Input: part model. Units: mm. Frame: model coordinates. Face numbers are marked on the shaded views. A direction names the side the tool comes from. Give positions to 0.01 mm unless a question says otherwise; leave off trailing zeros. Order: outer loops, then holes, each group sorted by start corner. A loop starts at its lowest first (then second) coordinate and runs counter-clockwise, first axis right, second up. Notation, with made-up numbers: (35.25, 29) - (48.25, 29) arc R25 ccw to (48.25, 55) - close; hole circle Ø7 at (5.5, 38.25). An arc over 180 degrees is marked (long way). Use a Markdown table: item, result.
Autodesk Inventor part; units mm, degrees
ref_plane "YZ Plane" through (0, 0, 0) normal (1, 0, 0) x (0, 1, 0)
ref_plane "XZ Plane" through (0, 0, 0) normal (0, 1, 0) x (-1, 0, 0)
ref_plane "XY Plane" through (0, 0, 0) normal (0, 0, 1) x (1, 0, 0)
sketch "Boceto1" plane through (0, 0, 0) normal (0, 1, 0) x (-1, 0, 0)
  line L0 (160, -36) -> (165, -36)
  line L1 (165, -36) -> (165, -101)
  line L2 (165, -101) -> (-5, -101)
  line L3 (160, 0) -> (0, 0)
  line L4 (0, 0) -> (0, -36)
  line L5 (0, -36) -> (-5, -36)
  line L6 (-5, -36) -> (-5, -101)
  line L7 (160, 0) -> (160, -36)
  dimension "d250" = 0
  dimension "d4" = 5
  dimension "d5" = 65
  dimension "d87" = 36
  dimension "d88" = 5
  dimension "d89" = 65
  dimension "d132" = 160
  dimension "d301" = 36
extrude "Extrusión1" add sketch "Boceto1" against normal blind 5
sketch "Boceto3" plane through (-160, 0, 0) normal (0, 0, 1) x (1, 0, 0)
  line L0 (0, 0) -> (160, 0)
  line L1 (160, -5) -> (0, -5)
  line L2 (80, -2.5) -> (80, -5)
  line L3 (160, -5) -> (80, -5)
  line L4 (80, -5) -> (100.5, -5)
  line L5 (100.5, -5) -> (100.5, -2.5)
  line L6 (100.5, -2.5) -> (59.5, -2.5)
  line L7 (59.5, -2.5) -> (59.5, -5)
  line L8 (59.5, -5) -> (80, -5)
  point P0 (100, -5)
  point P1 (60, -5)
  point P2 (165, -5)
  dimension "d140" = 80
  dimension "d410" = 20.5
  dimension "d411" = 2.5
  dimension "d412" = 41
  dimension "d413" = 2.5
extrude "Extrusión2" cut sketch "Boceto3" against normal blind 16
sketch "Boceto4" plane through (0, 0, 0) normal (0, 1, 0) x (1, 0, 0)
  circle A0 centre (-7.55, 15) radius 1.75
  circle A1 centre (-31.75, 15) radius 1.75
  circle A2 centre (-152.45, 15) radius 1.75
  circle A3 centre (-128.25, 15) radius 1.75
  line L0 (-140, 0) -> (-140, 36)
  line L1 (0, 0) -> (0, 15)
  line L2 (0, 36) -> (0, 0)
  line L3 (0, 15) -> (-7.55, 15)
  line L4 (-160, 0) -> (-160, 15)
  line L5 (-160, 0) -> (-160, 36)
  line L6 (-160, 15) -> (-152.45, 15)
  line L7 (-152.45, 15) -> (-128.25, 15)
  line L8 (-7.55, 15) -> (-31.75, 15)
  dimension "d16" = 3.5
  dimension "d18" = 3.5
  dimension "d21" = 3.5
  dimension "d23" = 3.5
  dimension "d138" = 15
  dimension "d141" = 7.55
  dimension "d142" = 15
  dimension "d143" = 7.55
extrude "Extrusión3" cut sketch "Boceto4" against normal blind 5
sketch "Boceto5" plane through (0, 0, 0) normal (0, 1, 0) x (1, 0, 0)
  line L0 (-165, 36) -> (-165, 101)
  line L1 (-165, 101) -> (5, 101)
  line L2 (-165, 36) -> (-160, 36)
  line L3 (-160, 41) -> (-160, 41)
  line L4 (-160, 41) -> (-160, 96)
  line L5 (-160, 96) -> (0.7104, 96)
  line L6 (-160, 41) -> (-160, 36)
  line L7 (-9.2896, 35) -> (-9.2896, 39.9954)
  line L8 (5, 36) -> (5, 101)
  line L9 (5, 101) -> (5, 36)
  line L10 (5, 36) -> (0, 36)
  line L11 (0, 36) -> (0, 96)
  point P0 (0, 0)
  point P1 (25, 35)
  dimension "d28" = 5
extrude "Extrusión4" add sketch "Boceto5" along normal blind 55
sketch "Boceto10" plane through (0, 0, 0) normal (0, 1, 0) x (1, 0, 0)
  line L0 (0, 0) -> (-80, 0)
  line L1 (0, 0) -> (-160, 0)
  line L2 (-80, 0) -> (-80, 60)
  line L3 (-80, 60) -> (-80, 42.5)
  line L4 (-80, 60) -> (-55, 60)
  ellipse E0 centre (-80, 60) end of major axis (-80, 42.5) minor radius 25
  point P0 (-60, 0)
  dimension "d74" = 80
  dimension "d75" = 60
  dimension "d76" = 17.5
  dimension "d77" = 25
extrude "Extrusión9" add sketch "Boceto10" along normal blind 3.3
sketch "Boceto11" plane through (0, 3.3, 0) normal (0, 1, 0) x (1, 0, 0)
  ellipse E0 centre (-80, 60) end of major axis (-55, 60) minor radius 17.5
  line L0 (-80, 60) -> (-60.5, 60)
  line L1 (-80, 60) -> (-99.5, 60)
  circle A0 centre (-80, 60) radius 15
  circle A1 centre (-99.5, 60) radius 2
  circle A2 centre (-60.5, 60) radius 2
  line L2 (0, 36) -> (0, 0)
  line L3 (-160, 0) -> (0, 0)
  dimension "d80" = 19.5
  dimension "d81" = 19.5
  dimension "d82" = 30
  dimension "d83" = 4
  dimension "d84" = 4
extrude "Extrusión10" cut sketch "Boceto11" against normal blind 15 contours L1 A0 L0 | L0 A0 L1 | A2 | A1
sketch "Boceto14" plane through (0, 0, 0) normal (0, 1, 0) x (1, 0, 0)
  line L0 (-160, 0) -> (0, 0)
  line L1 (-101.57, 13.86) -> (-58.43, 13.86)
  line L2 (-58.43, 35) -> (-101.57, 35)
  line L3 (-101.57, 35) -> (-101.57, 13.86)
  ellipse E0 centre (-80, 60) end of major axis (-55, 60) minor radius 17.5
  line L4 (-58.43, 35) -> (-58.43, 13.86)
  dimension "d328" = 21.14
  dimension "d375" = 43.14
extrude "Extrusión13" add sketch "Boceto14" along normal blind 5 contours L3 L2 L4 L1
sketch "Boceto15" plane through (0, 5, 0) normal (0, 1, 0) x (1, 0, 0)
  line L0 (-58.43, 35) -> (-101.57, 35)
  line L1 (-101.57, 35) -> (-95.07, 35)
  line L2 (-95.07, 35) -> (-95.07, 32.5)
  line L3 (-58.43, 13.86) -> (-64.93, 13.86)
  line L4 (-64.93, 13.86) -> (-64.93, 16.36)
  circle A0 centre (-95.07, 32.5) radius 1.5
  circle A1 centre (-64.93, 16.36) radius 1.5
  line L5 (-95.07, 32.5) -> (-64.93, 32.5)
  point P0 (0, 0)
  dimension "d158" = 6.5
  dimension "d159" = 2.5
  dimension "d160" = 6.5
  dimension "d161" = 2.5
  dimension "d162" = 3
  dimension "d163" = 3
extrude "Extrusión14" cut sketch "Boceto15" against normal blind 5
sketch "Boceto16" plane through (0, 5, 0) normal (0, 1, 0) x (1, 0, 0)
  line L0 (-58.43, 35) -> (-101.57, 35)
  line L1 (-58.43, 35) -> (-61.43, 35)
  line L2 (-61.43, 35) -> (-61.43, 13.86)
  line L3 (-61.43, 13.86) -> (-58.43, 13.86)
  line L4 (-58.43, 13.86) -> (-58.43, 35)
  line L5 (-98.57, 35) -> (-101.57, 35)
  line L6 (-101.57, 35) -> (-101.57, 13.86)
  line L7 (-101.57, 13.86) -> (-98.57, 13.86)
  line L8 (-98.57, 13.86) -> (-98.57, 35)
  point P0 (0, 0)
  dimension "d166" = 3
  dimension "d168" = 21.14
  dimension "d169" = 3
  dimension "d170" = 21.14
  dimension "d374" = 43.14
extrude "Extrusión15" cut sketch "Boceto16" against normal blind 5
sketch "Boceto17" plane through (0, 0, 0) normal (0, 1, 0) x (1, 0, 0)
  line L0 (0, 96) -> (-160, 96)
  line L1 (0, 96) -> (0, 86)
  line L2 (0, 36) -> (0, 96)
  line L3 (0, 86) -> (-13, 86)
  circle A0 centre (-13, 86) radius 3
  line L4 (-13, 86) -> (-49.54, 86)
  line L5 (-49.54, 86) -> (-49.54, 49.46)
  line L6 (-49.54, 49.46) -> (-13, 49.46)
  line L7 (-13, 49.46) -> (-13, 86)
  circle A1 centre (-49.54, 86) radius 3
  circle A2 centre (-49.54, 49.46) radius 3
  circle A3 centre (-13, 49.46) radius 3
  point P0 (0, 0)
  dimension "d173" = 10
  dimension "d174" = 13
  dimension "d175" = 6
  dimension "d176" = 36.54
  dimension "d177" = 36.54
  dimension "d178" = 36.54
  dimension "d182" = 6
  dimension "d183" = 6
  dimension "d184" = 6
extrude "Extrusión16" add sketch "Boceto17" along normal blind 4 contours A0 L7 L3 | L3 L4 A0 | L7 A0 L4 | A1 L5 L4 | L4 L5 A1 | A3 L6 L7 | L7 L6 A3 | A2 L6 L5 | L5 L6 A2
sketch "Boceto18" plane through (-49.54, 4, -86) normal (0, 1, 0) x (1, 0, 0)
  circle A0 centre (0, 0) radius 1.5
  circle A1 centre (36.54, 0) radius 3
  circle A2 centre (36.54, 0) radius 1.5
  circle A3 centre (0, -36.54) radius 3
  circle A4 centre (0, -36.54) radius 1.5
  circle A5 centre (36.54, -36.54) radius 3
  circle A6 centre (36.54, -36.54) radius 1.5
  point P0 (49.54, -86)
  dimension "d187" = 3
  dimension "d188" = 3
  dimension "d189" = 3
  dimension "d190" = 3
extrude "Extrusión17" cut sketch "Boceto18" against normal blind 5 contours A0 | A2 | A4 | A6
sketch "Boceto21" plane through (0, 55, 0) normal (0, 1, 0) x (1, 0, 0)
  circle A0 centre (5, 40) radius 4
  line L0 (-165, 36) -> (-165, 101)
  circle A1 centre (-165, 96) radius 4
  circle A2 centre (-165, 40) radius 4
  line L1 (0, 96) -> (-160, 96)
  line L2 (0, 96) -> (5, 96)
  circle A3 centre (5, 96) radius 4
  line L3 (-165, 101) -> (-165, 96)
  point P0 (0, 0)
  point P1 (-165, 41.5)
  point P2 (-165, 38.5)
  point P3 (5, 101)
  dimension "d210" = 8
  dimension "d214" = 8
  dimension "d215" = 8
  dimension "d262" = 5
  dimension "d263" = 8
  dimension "d372" = 5
extrude "Extrusión18" add sketch "Boceto21" against normal blind 10
sketch "Boceto22" plane through (0, 55, 0) normal (0, 1, 0) x (1, 0, 0)
  arc A0 (5, 36) -> (5, 44) centre (5, 40) ccw
  arc A1 (5, 91.0001) -> (5, 98.9999) centre (4.9732, 95) ccw
  arc A2 (-165, 100) -> (-165, 92) centre (-165, 96) ccw
  circle A3 centre (-165, 96) radius 1.5
  line L0 (-165, 36) -> (-165, 101)
  circle A4 centre (-165, 40) radius 1.5
  line L1 (0, 96) -> (0, 36)
  circle A5 centre (5, 96) radius 1.5
  line L2 (5, 40) -> (0, 40)
  line L3 (0, 36) -> (0, 40)
  circle A6 centre (5, 40) radius 1.5
  line L4 (0, 96) -> (5, 96)
  line L5 (-160, 96) -> (-160, 36)
  point P0 (0, 0)
  dimension "d218" = 3
  dimension "d219" = 3
  dimension "d259" = 3
  dimension "d260" = 5
  dimension "d261" = 3
extrude "Extrusión19" cut sketch "Boceto22" against normal blind 5 contours A4 L0 | L0 A4 | L0 A3 | A3 L0 | A6 | A5
sketch "Boceto24" plane through (-160, 0, -96) normal (0, 0, 1) x (1, 0, 0)
  line L0 (0, 55) -> (160, 55)
  line L1 (29.2, 0) -> (0, 0)
  line L2 (0, 0) -> (29.2, 0)
  line L3 (0, 0) -> (0, -5)
  line L4 (0, 0) -> (0, 41)
  line L5 (0, 0) -> (0, 55)
  line L6 (0, 41) -> (29.2, 41)
  line L7 (29.2, 41) -> (29.2, 0)
  line L8 (29.2, 0) -> (0, 0)
  line L9 (32.2, 44) -> (-3, 44)
  line L10 (-3, 44) -> (-3, -3)
  line L11 (-3, -3) -> (32.2, -3)
  line L12 (32.2, -3) -> (32.2, 44)
  line L13 (29.2, 0) -> (29.2, 10)
  line L14 (29.2, 10) -> (0, 10)
  point P0 (160, 0)
  point P1 (0, 10)
  point P2 (0, 44)
  point P3 (0, -3)
  dimension "d243" = 41
  dimension "d244" = 29.2
  dimension "d246" = 3
  dimension "d247" = 10
  dimension "d248" = 29.2
extrude "Extrusión21" cut sketch "Boceto24" against normal blind 10 contours L14 L4 L6 L7
extrude "Extrusión22" add sketch "Boceto24" along normal blind 61 contours L7 L6 L5 L9 L12 L11 L3 L1
sketch "Boceto25" plane through (-160, 44, -96) normal (0, 1, 0) x (1, 0, 0)
  line L0 (0, -96) -> (0, -60)
  line L1 (0, -61) -> (0, -64)
  line L2 (0, -64) -> (32.2, -64)
  line L3 (32.2, -64) -> (32.2, -61)
  line L4 (32.2, -61) -> (0, -61)
  point P0 (160, -96)
  point P1 (0, -61)
extrude "Extrusión23" add sketch "Boceto25" against normal blind 44
sketch "Boceto26" plane through (5, -5, -101) normal (0, 0, -1) x (-1, 0, 0)
  line L0 (125.8, 46) -> (125.8, 31)
  line L1 (125.8, 31) -> (120.8, 31)
  line L2 (132.8, 49) -> (132.8, 5)
  line L3 (120.8, 31) -> (130.8, 31)
  line L4 (130.8, 31) -> (130.8, 13)
  line L5 (130.8, 13) -> (120.8, 13)
  line L6 (120.8, 13) -> (120.8, 31)
  line L7 (135.8, 46) -> (135.8, 5)
  line L8 (125.8, 46) -> (135.8, 46)
  point P0 (5, 5)
  dimension "d277" = 15
  dimension "d278" = 5
  dimension "d280" = 18
  dimension "d281" = 10
extrude "Extrusión24" add sketch "Boceto26" along normal blind 12
sketch "Boceto28" plane through (-125.8, 8, -101) normal (-1, 0, 0) x (0, 0, 1)
  line L0 (-12, 0) -> (-12, 9)
  line L1 (-12, 0) -> (-12, 18)
  line L2 (-12, 9) -> (-6, 9)
  line L3 (-9.5, 1.5) -> (-2.5, 1.5)
  line L4 (-2.5, 1.5) -> (-2.5, 16.5)
  line L5 (-2.5, 16.5) -> (-9.5, 16.5)
  line L6 (-9.5, 16.5) -> (-9.5, 1.5)
  point P0 (101, -8)
  dimension "d293" = 9
  dimension "d294" = 6
  dimension "d297" = 7
  dimension "d298" = 15
extrude "Extrusión25" cut sketch "Boceto28" against normal blind 10
sketch "Boceto31" plane through (0, 0, 0) normal (0, 1, 0) x (1, 0, 0)
  circle A0 centre (-69, 6) radius 2
  circle A1 centre (-91, 6) radius 2
  line L0 (-91, 6) -> (-69, 6)
  line L1 (-80, 0) -> (-80, 6)
  point P0 (0, 0)
  dimension "d368" = 4
  dimension "d369" = 4
  dimension "d376" = 6
extrude "Extrusión30" cut sketch "Boceto31" against normal blind 5
sketch "Boceto33" plane through (5, -5, -101) normal (0, 0, -1) x (-1, 0, 0)
  line L0 (120.8, 31) -> (130.8, 31)
  line L1 (125.8, 31) -> (125.8, 36)
  line L2 (125.8, 36) -> (123.19, 36)
  line L3 (125.8, 36) -> (128.41, 36)
  line L4 (128.41, 36) -> (128.41, 46.22)
  line L5 (128.41, 46.22) -> (123.19, 46.22)
  line L6 (123.19, 46.22) -> (123.19, 36)
  line L7 (120.19, 49.22) -> (131.41, 49.22)
  line L8 (131.41, 49.22) -> (131.41, 33)
  line L9 (131.41, 33) -> (125.8, 33)
  line L10 (125.8, 33) -> (120.19, 33)
  line L11 (120.19, 33) -> (120.19, 49.22)
  point P0 (5, 5)
  dimension "d387" = 5
  dimension "d388" = 2.61
  dimension "d389" = 2.61
  dimension "d390" = 10.22
  dimension "d391" = 5.22
  dimension "d394" = 3
extrude "Extrusión34" add sketch "Boceto33" against normal blind 10.7
extrude "Extrusión35" cut sketch "Boceto33" against normal blind 8.7 contours L2 L6 L5 L4 L3
properties part number "Mitad_2"
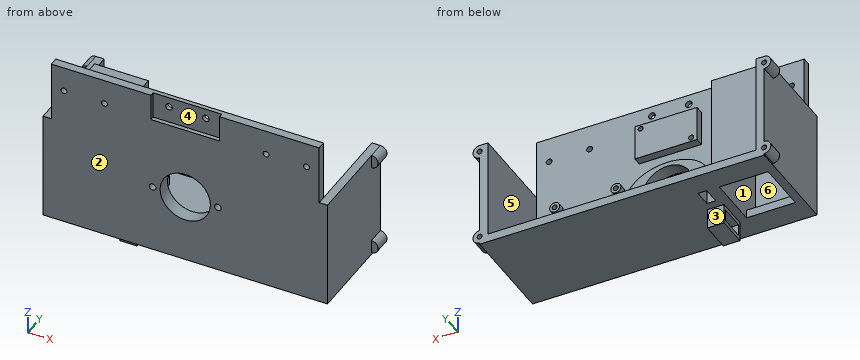
1. Pin query (flat end, axial travel): pin 1 (5 mm diameter, centred on x = -74, z = -75, fed in from +Y); pin 2 (5.5 mm diameter, centred on x = -152.45, z = -15, fed in from +Y); pin 3 (5 mm diameter, centred on x = -14, z = -85, fed in from +Y); pin 4 (2.5 mm diameter, centred on x = -99.5, z = -60, fed in from -Y). Return the tip coordinate at first contact, or that it passes through.
Response:
| item | result |
|---|---|
| pin 1 | stops at y = 3.3 |
| pin 2 | stops at y = 0 |
| pin 3 | stops at y = 4 |
| pin 4 | passes through |
2. Mould query, pull axis Z, two halves, no side actions, for the marked faces 1 and 2. Classes: pulls with the +Z half, pulls with the -Z half, needs draft (parallel to the pull), parting line crosses it, or undercut.
Response:
| item | result |
|---|---|
| face 1 | undercut |
| face 2 | needs draft |
3. Section query A-A (z = -80.5). Return loops of the section in (x, y).
Response:
| item | result |
|---|---|
| outline | (-165, -5) - (5, -5) - (5, 55) - (0, 55) - (0, 0) - (-127.8, 0) - (-127.8, 44) - (-160, 44) - (-160, 55) - (-165, 55) - close; hole (-160, 0) - (-130.8, 0) - (-130.8, 41) - (-160, 41) - close |
4. Section query D-D (x = -69). State how many separate pieces and enclosed holes the cut face has, then the cut area to 3 significant figures.
Response:
| item | result |
|---|---|
| separate pieces | 3 |
| enclosed holes | 0 |
| area | 770 mm^2 |
5. Material intervals for line 1 along Z through (x, y) = (-13, 0.5); line 2 along X through (y, z) = (35, -95.5); line 3 along X through (y, z) = (21, -77), sorted ascending.
Response:
| item | result |
|---|---|
| line 1 | z = -101 to -96, -89 to -87.5, -84.5 to -83, -52.46 to -50.96, -47.96 to -46.46 |
| line 2 | x = -165 to -160, -130.8 to -127.8, -126.41 to -123.41, -118.19 to -115.19, 0 to 5 |
| line 3 | x = -165 to -160, -130.8 to -127.8, 0 to 5 |
6. Section query B-B (y = 14.5). Return loops of the section in (x, z), then the cut area to 3 significant figures.
Response:
| item | result |
|---|---|
| outline | (-165, -101) - (-160, -101) - (-160, -36) - (-165, -36) - close; (-160, -35) - (-130.8, -35) - (-130.8, -101) - (-125.8, -101) - (-125.8, -103.5) - (-115.8, -103.5) - (-115.8, -101) - (5, -101) - (5, -36) - (0, -36) - (0, -96) - (-127.8, -96) - (-127.8, -32) - (-160, -32) - close; (-125.8, -113) - (-115.8, -113) - (-115.8, -110.5) - (-125.8, -110.5) - close |
| area | 1,630 mm^2 |
7. Set-up query: the marked faces 3, 4, 5 and 6. Return all of +Z, -Z, +X, -X, +Y, -Y with unobstructed straight access to the full face (end or side cutting, diameter ignored); none if empty.
Response:
| item | result |
|---|---|
| face 3 | -Z, +X, -X, +Y |
| face 4 | +Z, -Y |
| face 5 | +Z, +Y |
| face 6 | none |
8. Section query C-C (x = -108.5). Return loops of the section in (y, z).
Response:
| item | result |
|---|---|
| outline | (-5, -101) - (55, -101) - (55, -96) - (0, -96) - (0, 0) - (-5, 0) - close |
